from build123d import *

# Parameters (mm, degrees)
F1_DEPTH = 20
F2_R     = 32.5
F3_DEPTH = 158
F4_W     = 125.283194
F4_H     = 69.601772
F5_DEPTH = 25


with BuildPart() as f1:
    # F0 (on Front) → F1 (new body)
    with BuildSketch(Plane.XZ):
        with BuildLine():
            ThreePointArc((62.641597, 27.300886), (67.944897, 40.104186), (55.141597, 34.800886))
            Line((55.141597, 34.800886), (-55.141597, 34.800886))
            ThreePointArc((-55.141597, 34.800886), (-67.944897, 40.104186), (-62.641597, 27.300886))
            Line((-62.641597, 27.300886), (-62.641597, -27.300886))
            ThreePointArc((-62.641597, -27.300886), (-67.944897, -40.104186), (-55.141597, -34.800886))
            Line((-55.141597, -34.800886), (55.141597, -34.800886))
            ThreePointArc((55.141597, -34.800886), (67.944897, -40.104186), (62.641597, -27.300886))
            Line((62.641597, -27.300886), (62.641597, 27.300886))
        make_face()
    extrude(amount=F1_DEPTH)

    # F2 (on face) → F3 (join)
    with BuildSketch(Plane.XZ.offset(20)):
        Circle(F2_R)
    extrude(amount=F3_DEPTH)

    # F4 (on face) → F5 (join)
    with BuildSketch(Plane.XZ.offset(178)):
        Rectangle(F4_W, F4_H)
    extrude(amount=F5_DEPTH)


solid = f1.part
Input: part model. Units: mm. Frame: model coordinates. A direction names the side the tool comes from. Round coordinates to 2 decimals unless told otherwise and drop trailing zeros. Write each loop counter-clockwise with the first axis right and the second up, starting at its lowest first coordinate (ties: lowest second). Pieces come first, ordered by that corner, then holes.
1) Contact query for flat-ended pins moving along their axis: P1, Ø6, axis at y = -7, z = -7, coming from the +X side; P2, Ø5, axis at x = 21, z = -4, coming from the +Y side; P3, Ø1.5, axis at y = -155.5, z = 27, coming from the -X side; P4, Ø10, axis at x = 15, y = -9, coming from the -Z side. Output: stop coordinate, or through.
2) Cut plane C-C (y = -15). Return the cut outline in (x, z), then the cut area to 3 significant figures.
3) Ray query, L1, parallel to Y at x = 46, z = 33.5; L2, parallel to X at y = -9, z = 23; L3, parallel to Z at x = 10.5, y = -12. Return the intervals inside material, ascending.
4) Draft query along X for faces 6 (the cylindrical face through (67.767, -9.86, -40.276)), 7 (the flat face through (-62.642, -10, 0)), 8 (the flat face through (-29, -178, 16)). Return one class per face: pulls with the +X half, pulls with the -X half, needs draft (parallel to the pull), parting line crosses it, or undercut.
5) Cut plane D-D (x = -6). Return the cut outline in (y, z).
6) Reachability of faces 1 (the flat face through (62.642, -10, 0)), 2 (the flat face through (-1, -10, -34.801)), 3 (the flat face through (-62.642, -190, 0)), 4 (the cylindrical face through (31, -97.89, 9.76)), 5 (the flat face through (1, -10, 34.801)) from +Z, -Z, +X, -X, +Y, -Y: full face, straight path, thin tool, end or side. Return the list, or none.
7) Cut plane A-A (x = 39.5). Return the cut outline in (y, z), then the cut area to 3 significant figures.
8) Cut plane B-B (z = -12.5). Return the cut outline in (x, y).
Geometry says:
1. P1: stops at x = 62.64
1. P2: stops at y = 0
1. P3: stops at x = -19.16
1. P4: stops at z = -34.8
2. outline: (-62.64, -27.3) arc R7.5 ccw (long way) to (-55.14, -34.8) - (55.14, -34.8) arc R7.5 ccw (long way) to (62.64, -27.3) - (62.64, 27.3) arc R7.5 ccw (long way) to (55.14, 34.8) - (-55.14, 34.8) arc R7.5 ccw (long way) to (-62.64, 27.3) - close
2. area: 9,250 mm2
3. L1: y = -203 to -178, -20 to 0
3. L2: x = -62.64 to 62.64
3. L3: z = -34.8 to 34.8
4. face 6: undercut
4. face 7: pulls with the -X half
4. face 8: needs draft
5. outline: (-203, -34.8) - (-178, -34.8) - (-178, -31.94) - (-20, -31.94) - (-20, -34.8) - (0, -34.8) - (0, 34.8) - (-20, 34.8) - (-20, 31.94) - (-178, 31.94) - (-178, 34.8) - (-203, 34.8) - close
6. face 1: +X, +Y, -Y
6. face 2: -Z, +Y, -Y
6. face 3: +Z, -Z, -X, -Y
6. face 4: none
6. face 5: +Z, +Y, -Y
7. outline: (-203, -34.8) - (-178, -34.8) - (-178, 34.8) - (-203, 34.8) - close; (-20, -34.8) - (0, -34.8) - (0, 34.8) - (-20, 34.8) - close
7. area: 3,130 mm2
8. outline: (-62.64, -203) - (62.64, -203) - (62.64, -178) - (30, -178) - (30, -20) - (62.64, -20) - (62.64, 0) - (-62.64, 0) - (-62.64, -20) - (-30, -20) - (-30, -178) - (-62.64, -178) - close
